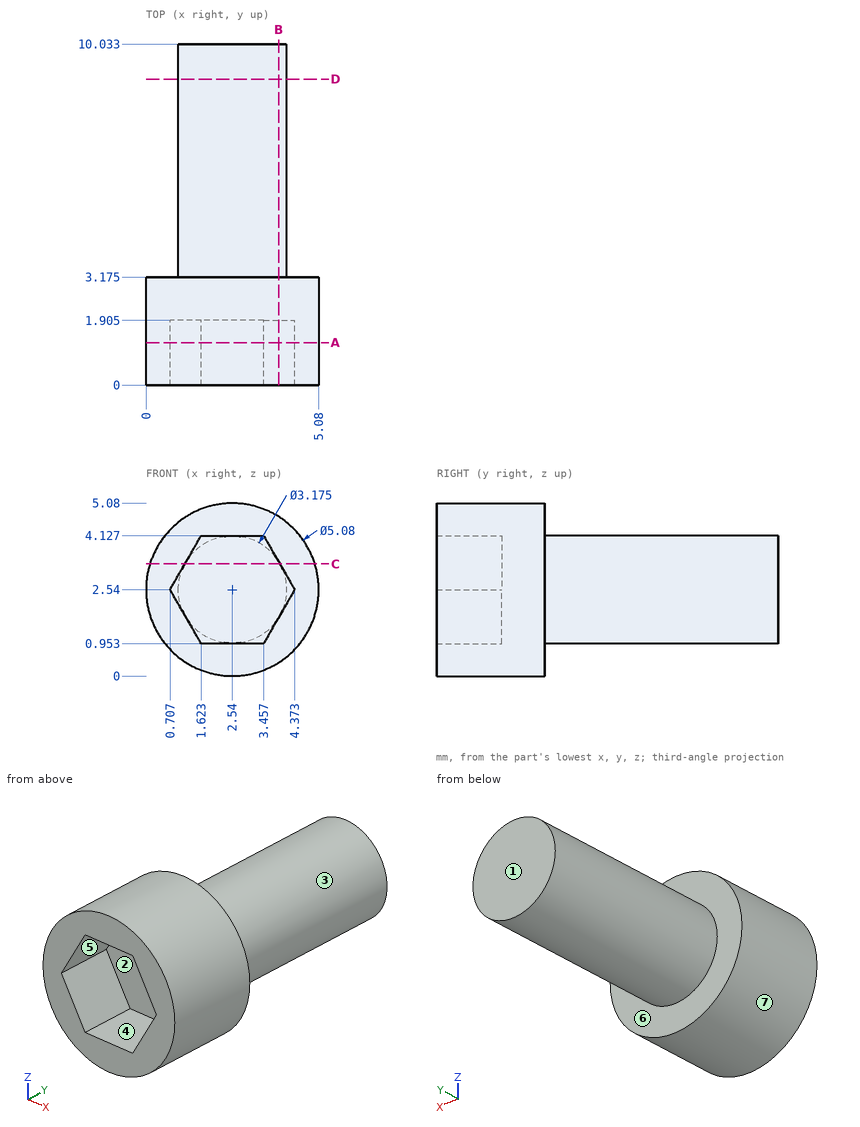
Input: dimensioned drawing with shaded views. Units: mm. Origin: part minimum x, y, z. A direction names the side the tool comes from. Round coordinates to 2 decimals unless told otherwise and drop trailing zeros. Order: outer loops, then holes, each group sorted by start corner. A loop starts at its lowest first (then second) coordinate and runs counter-clockwise, first axis right, second up.
1. Cut plane D-D, the plane y = 9. Output: boundary loops of the cut face in (x, z) (1 decimal).
The answers:
outline: circle Ø3.2 at (2.5, 2.5)
2. Mould query, pull axis Z, two halves, no side actions, for the marked faces 4, 5, 6 and 7. Classes: released by +Z, released by -Z, zero draft, split by the parting line, or undercut.
The answers:
face 4: undercut
face 5: undercut
face 6: zero draft
face 7: split by the parting line
3. Pin query (flat end, axial travel): P1, Ø2, axis at x = 4.5, y = 5.5, coming from the -Z side (1 decimal); P2, Ø1, axis at x = 2.5, z = 3, coming from the -Y side (1 decimal); P3, Ø1, axis at x = 3, y = 7, coming from the -Z side. Return the tip coordinate at first contact, or that it passes through.
The answers:
P1: stops at z = 1.3
P2: stops at y = 1.9
P3: stops at z = 0.95
4. Cut plane C-C, the plane z = 3.3. Output: boundary loops of the cut face in (x, y) (1 decimal), then the cut area to 3 significant figures.
The answers:
outline: (0.1, 0) - (1.1, 0) - (1.1, 1.9) - (3.9, 1.9) - (3.9, 0) - (5, 0) - (5, 3.2) - (3.9, 3.2) - (3.9, 10) - (1.1, 10) - (1.1, 3.2) - (0.1, 3.2) - close
area: 29.2 mm2
5. Set-up query: the marked faces 1, 2 and 3. Return all of +Z, -Z, +X, -X, +Y, -Y with unobstructed straight access to the full face (end or side cutting, diameter ignored); none if empty.
The answers:
face 1: +Z, -Z, +X, -X, +Y
face 2: -Y
face 3: +Y
6. Cut plane B-B, the plane x = 3.9. Output: boundary loops of the cut face in (y, z) (1 decimal).
The answers:
outline: (0, 0.4) - (3.2, 0.4) - (3.2, 1.7) - (10, 1.7) - (10, 3.4) - (3.2, 3.4) - (3.2, 4.7) - (0, 4.7) - (0, 3.4) - (1.9, 3.4) - (1.9, 1.7) - (0, 1.7) - close
7. Cut plane A-A, the plane y = 1.25. Output: boundary loops of the cut face in (x, z).
The answers:
outline: circle Ø5.08 at (2.54, 2.54); hole (0.71, 2.54) - (1.62, 0.95) - (3.46, 0.95) - (4.37, 2.54) - (3.46, 4.13) - (1.62, 4.13) - close
8. Material intervals for line 1 (Y direction, x = 1.25, z = 1) (1 decimal); line 2 (Y direction, x = 2.6, z = 1.6) (1 decimal); line 3 (X direction, y = 7.75, z = 2.55), sorted ascending.
The answers:
line 1: y = 0 to 3.2
line 2: y = 1.9 to 10
line 3: x = 0.95 to 4.13
